```python
from build123d import *

# Parameters (mm, degrees)
SKETCH1_W           = 500
SKETCH1_H           = 400
SKETCH1_R           = 1.5
SKETCH1_R_2         = 1.525
BOSS_EXTRUDE1_DEPTH = 6
SKETCH2_R           = 1.5
CUT_EXTRUDE1_DEPTH  = 10
SKETCH3_W           = 50
SKETCH3_H           = 60
SKETCH3_R           = 7.5
CUT_EXTRUDE2_DEPTH  = 7
FILLET1_R           = 10
BOSS_EXTRUDE2_START = -6
SKETCH4_W           = 6
SKETCH4_H           = 400
BOSS_EXTRUDE2_DEPTH = 6


with BuildPart() as part:
    # Sketch1 → Boss-Extrude1 (new body)
    with BuildSketch(Plane(origin=(0, 0, 0), x_dir=(1, 0, 0), z_dir=(0, 1, 0))):
        with Locations((250, -200)):
            Rectangle(SKETCH1_W, SKETCH1_H)
        with Locations((490, -378)):
            Circle(SKETCH1_R, mode=Mode.SUBTRACT)
        with Locations((10, -378)):
            Circle(SKETCH1_R, mode=Mode.SUBTRACT)
        with Locations((236.4, -195.2)):
            Circle(SKETCH1_R, mode=Mode.SUBTRACT)
        with Locations((262.1, -195.2)):
            Circle(SKETCH1_R, mode=Mode.SUBTRACT)
        with Locations((262.1, -142.9)):
            Circle(SKETCH1_R, mode=Mode.SUBTRACT)
        with Locations((236.4, -142.9)):
            Circle(SKETCH1_R, mode=Mode.SUBTRACT)
        with Locations((8, -21.5)):
            Circle(SKETCH1_R, mode=Mode.SUBTRACT)
        with Locations((488, -21.5)):
            Circle(SKETCH1_R_2, mode=Mode.SUBTRACT)
    extrude(amount=BOSS_EXTRUDE1_DEPTH)

    # Sketch2 → Cut-Extrude1 (cut)
    with BuildSketch(Plane(origin=(0, 6, 0), x_dir=(1, 0, 0), z_dir=(0, 1, 0))):
        with Locations((165, -378)):
            Circle(SKETCH2_R)
        with Locations((165, -392)):
            Circle(SKETCH2_R)
        with Locations((335, -378)):
            Circle(SKETCH2_R)
        with Locations((335, -392)):
            Circle(SKETCH2_R)
    extrude(amount=-CUT_EXTRUDE1_DEPTH, mode=Mode.SUBTRACT)

    # Sketch3 → Cut-Extrude2 (cut, through all)
    with BuildSketch(Plane.XZ):
        with Locations((275, 370)):
            Rectangle(SKETCH3_W, SKETCH3_H)
        with Locations((225, 370)):
            Rectangle(SKETCH3_W, SKETCH3_H)
        with Locations((250, 240)):
            Circle(SKETCH3_R)
    extrude(amount=-CUT_EXTRUDE2_DEPTH, mode=Mode.SUBTRACT)

    # Fillet1
    fillet1_edges = [part.edges().sort_by_distance(p)[0] for p in [
        (300, 3, 340),
        (200, 3, 340),
        (200, 3, 400),
        (300, 3, 400),
    ]]
    fillet(fillet1_edges, radius=FILLET1_R)

    # Sketch4 → Boss-Extrude2 (add)
    with BuildSketch(Plane.XZ.offset(BOSS_EXTRUDE2_START)):
        with Locations((-3, 200)):
            Rectangle(SKETCH4_W, SKETCH4_H)
        with Locations((503, 200)):
            Rectangle(SKETCH4_W, SKETCH4_H)
    extrude(amount=BOSS_EXTRUDE2_DEPTH)


solid = part.part
```
Model file for the job. Use its own axes, mm. A direction names the side the tool comes from. Coordinates: 2 decimals unless noted, no trailing zeros. Loops run counter-clockwise (first coordinate to the right, second up) from the corner with the lowest first, then second, coordinate; pieces in that order, holes last. Notation, with made-up numbers: (50.5, -7) - (101.5, -7) arc R20 cw to (101.5, 28) - close; hole circle Ø1 at (83, 26). An arc over 180 degrees is marked (long way). Answer as a JSON object with one key per item and string values. Group by question number.
(1) Tool access for faces 1 (the face through (303.01, 3.04, 397.15)), 2 (the face through (254.032, 2.958, 246.324)): list every direction of +Z, -Z, +X, -X, +Y, -Y with a clear straight run to the whole face (end or side of a thin tool).
(2) Cut at A-A (y = 2.65). State how many separate pieces and enclosed holes the cut face has, then the cut area to 3 significant figures.
(3) Two-plate mould, pull along X, no slides. Class faces 3 (the face through (297.15, 3.04, 343.01)), 4 (the face through (246, 6, 203)): released by +X, released by -X, zero draft, split by the parting line, or undercut.
(4) Cut at B-B (x = 250). Give the cut face in (y, z).
(5) Probe line 1 along X through (y, z) = (1.2, 378); line 2 along Z through (x, y) = (335, 3.4); line 3 along Z through (x, y) = (488, 2.5) (3 decimals). List the from-to ranges inside material, lowest first.
(6) Cut at C-C (z = 240). Give the cut face in (x, y).
(7) Flat gauge pin, fed straight in: pin 1 (1.8 mm diameter, centred on x = 236.4, z = 195.2, fed in from +Y). Where does the tip first touch, or does it go through?
Geometry says:
{
 "1": {"face 1": "+Z, +Y, -Y", "face 2": "+Y, -Y"},
 "2": {"separate pieces": "1", "enclosed holes": "13", "area": "199,000 mm^2"},
 "3": {"face 3": "undercut", "face 4": "zero draft"},
 "4": {"outline": "(0, 0) - (6, 0) - (6, 232.5) - (0, 232.5) - close; (0, 247.5) - (6, 247.5) - (6, 340) - (0, 340) - close"},
 "5": {"line 1": "x = -6 to 8.5, 11.5 to 163.5, 166.5 to 200, 300 to 333.5, 336.5 to 488.5, 491.5 to 506", "line 2": "z = 0 to 376.5, 379.5 to 390.5, 393.5 to 400", "line 3": "z = 0 to 19.975, 23.025 to 400"},
 "6": {"outline": "(-6, 0) - (242.5, 0) - (242.5, 6) - (-6, 6) - close; (257.5, 0) - (506, 0) - (506, 6) - (257.5, 6) - close"},
 "7": {"pin 1": "passes through"}
}
